from build123d import *

# Parameters (mm, degrees)
F0_W      = 32
F0_H      = 28
F0_R      = 1.6
F1_DEPTH  = 9.5
F3_DEPTH  = 4.5
F5_DEPTH  = 5
F8_R      = 2.6
F9_DEPTH  = 25
F11_DEPTH = 3
F12_R     = 3.1
F13_DEPTH = 3
F15_DEPTH = 25
F17_DEPTH = 10
F18_W     = 7.420289278
F18_H     = 10
F19_DEPTH = 5
F21_DEPTH = 25
F22_SIZE  = 1


with BuildPart() as f1:
    # F0 (on Front) → F1 (new body)
    with BuildSketch(Plane.XZ):
        Rectangle(F0_W, F0_H)
        with Locations((-10, 0)):
            Circle(F0_R, mode=Mode.SUBTRACT)
    extrude(amount=F1_DEPTH)

    # F2 (on face) → F3 (cut)
    with BuildSketch(Plane.XZ.offset(9.5)):
        Polygon((16, -14), (16, 14), (-6, 14), (2, 0), (-6, -14), align=None)
    extrude(amount=-F3_DEPTH, mode=Mode.SUBTRACT)

    # F4 (on face) → F5 (cut, through all)
    with BuildSketch(Plane.XZ.offset(5)):
        with BuildLine():
            Line((10.5927268367, 6), (-0.4072731633, 6))
            ThreePointArc((-0.4072731633, 6), (-4.516718781, 9.8971730932), (-10, 11.314610385))
            Line((-10, 11.314610385), (-20, 11.314610385))
            Line((-20, 11.314610385), (-20, -11.314610385))
            Line((-20, -11.314610385), (-10, -11.314610385))
            ThreePointArc((-10, -11.314610385), (-4.516718781, -9.8971730932), (-0.4072731633, -6))
            Line((-0.4072731633, -6), (10.5927268367, -6))
            Line((10.5927268367, -6), (10.5927268367, 6))
        make_face()
    extrude(amount=-F5_DEPTH, mode=Mode.SUBTRACT)

    # F7: F1 across plane


with BuildPart() as f1_1:
    add(f1.part)
    add(f1.part.mirror(Plane.XZ))

    # F8 (on face) → F9 (cut)
    with BuildSketch(Plane.YZ.offset(16)):
        Circle(F8_R)
    extrude(amount=-F9_DEPTH, mode=Mode.SUBTRACT)

    # F10 (on face) → F11 (cut)
    with BuildSketch(Plane(origin=(0, 9.5, 0), x_dir=(-1, 0, 0), z_dir=(0, 1, 0))):
        Polygon((10.1159347913, -3.2888537706), (12.9061983103, -1.5440244109), (12.790263519, 1.7448293597), (9.8840652087, 3.2888537706), (7.0938016897, 1.5440244109), (7.209736481, -1.7448293597), align=None)
    extrude(amount=-F11_DEPTH, mode=Mode.SUBTRACT)

    # F12 (on face) → F13 (cut)
    with BuildSketch(Plane.XZ.offset(9.5)):
        with Locations((-10, 0)):
            Circle(F12_R)
    extrude(amount=-F13_DEPTH, mode=Mode.SUBTRACT)

    # F14 (on face) → F15 (cut)
    with BuildSketch(Plane.XZ.offset(5)):
        Polygon((16, 6.8564745598), (16, 14), (-6, 14), align=None)
        Polygon((16, -6.8564745598), (-6, -14), (16, -14), align=None)
    extrude(amount=-F15_DEPTH, mode=Mode.SUBTRACT)

    # F16 (on face) → F17 (join, through all)
    with BuildSketch(Plane.XZ.offset(5)):
        Polygon((10.5927268367, 6), (4.4333031224, 6), (10.5927268367, 4), align=None)
        Polygon((4.4333031224, -6), (10.5927268367, -6), (10.5927268367, -4), align=None)
    extrude(amount=-F17_DEPTH)

    # F18 (on face) → F19 (cut)
    with BuildSketch(Plane.XY.offset(14)):
        with Locations((-12.289855361, 0)):
            Rectangle(F18_W, F18_H)
    extrude(amount=-F19_DEPTH, mode=Mode.SUBTRACT)

    # F20 (on face) → F21 (cut)
    with BuildSketch(Plane.XZ.offset(9.5)):
        Polygon((-16, 6.579710722), (-8.579710722, 14), (-16, 14), align=None)
    extrude(amount=-F21_DEPTH, mode=Mode.SUBTRACT)

    # F22
    f22_edges = [f1_1.edges().sort_by_distance(p)[0] for p in [
        (-8.579711, -5, 12.612557),
        (-8.579711, 5, 12.612557),
    ]]
    chamfer(f22_edges, length=F22_SIZE)


solid = f1_1.part
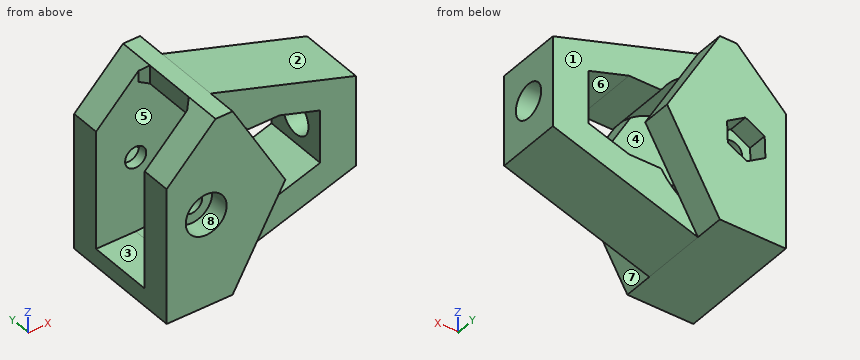
Check sheet for the modelled part. Datum: model origin and axes. Units: mm. Face numbers are marked on the shaded views. A direction names the side the tool comes from. Round coordinates to 2 decimals unless told otherwise and drop trailing zeros. Loops run counter-clockwise (first coordinate to the right, second up) from the corner with the lowest first, then second, coordinate; pieces in that order, holes last. Notation, with made-up numbers: M -36.75,27 L -25.75,27 A12 cw -25.75,35 Z; hole C 26,32 d4. An arc over 180 degrees is marked long. One line per item, written item: value.
(1) Depth check by flat-ended pin: pin 1 Ø6.5 at (x, z) = (8.5, 6) entering from -Y; pin 2 Ø4 at (x, y) = (0, 6) entering from +Z; pin 3 Ø2.5 at (y, z) = (-1, 1) entering from -X. Enter the tip coordinate at first touch or a pass-through.
Computed values:
pin 1: stops at y = -5
pin 2: stops at z = 12.61
pin 3: stops at x = 10.59
(2) Sectioned sample at B-B, the plane z = 0.5. Count the separate pieces of the cut face and the enclosed holes in it, then the cut area to 3 significant figures.
Computed values:
separate pieces: 6
enclosed holes: 0
area: 141 mm^2
(3) Sectioned sample at A-A, the plane y = 0. Record the cut outline in (x, z).
Computed values:
outline: M -16,-14 L -6,-14 L 16,-6.86 L 16,-2.6 L 10.59,-2.6 L 10.59,-4 L 4.43,-6 L -0.41,-6 A11.31 cw -10,-11.31 L -16,-11.31 Z; M -8.58,11.23 A11.31 cw -0.41,6 L 4.43,6 L 10.59,4 L 10.59,2.6 L 16,2.6 L 16,6.86 L -6,14 L -8.58,14 Z
(4) Sectioned sample at C-C, the plane x = 3. Record the cut outline in (y, z), then the cut area to 3 significant figures.
Computed values:
outline: M -5,-11.08 L 5,-11.08 L 5,-6 L -5,-6 Z; M -5,6 L 5,6 L 5,11.08 L -5,11.08 Z
area: 102 mm^2
(5) Thickness scan on line 1 (Y direction, x = -11.5, z = 6); line 2 (X direction, y = -6.05, z = 0); line 3 (Y direction, x = 3.5, z = -9.25). Record the ranges inside material, lowest first.
Computed values:
line 1: y = -9.5 to -5, 5 to 9.5
line 2: x = -16 to -11.6, -8.4 to 2
line 3: y = -5 to 5
(6) Release check for a two-part mould opening along Y. For the marked faces 1, 2, 3 and 4 record: +Y half, -Y half, draft (parallel to the pull), parting line (faces both ways), or undercut.
Computed values:
face 1: +Y half
face 2: draft
face 3: undercut
face 4: undercut
(7) Sectioned sample at D-D, the plane x = 14.5. Record the cut outline in (y, z), then the cut area to 3 significant figures.
Computed values:
outline: M -5,-7.34 L 5,-7.34 L 5,7.34 L -5,7.34 Z; hole C 0,0 d5.2
area: 126 mm^2
(8) Access from +Z, -Z, +X, -X, +Y, -Y to the whole of each face (thin tool, end or side, straight path). Record for the marked faces 5, 6, 7 and 8.
Computed values:
face 5: -X
face 6: -X, +Y, -Y
face 7: -Z, +X, -Y
face 8: -Y
